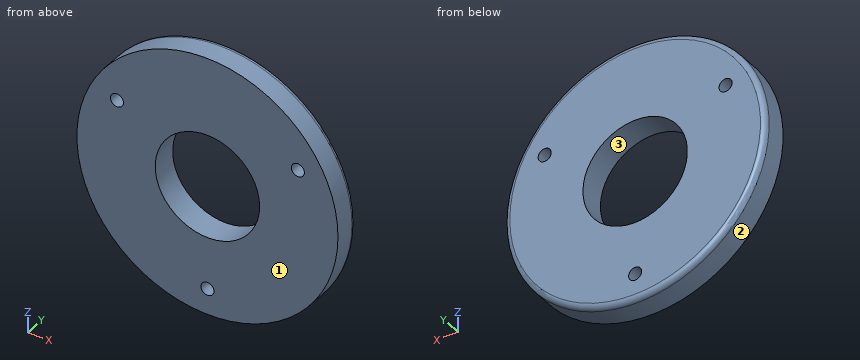
```python
from build123d import *

# Parameters (mm, degrees)
SKETCH1_R           = 63.5
BOSS_EXTRUDE1_DEPTH = 12.7
SKETCH2_R           = 25.4
CUT_EXTRUDE1_DEPTH  = 13.7
SKETCH3_R           = 3.175
CUT_EXTRUDE2_DEPTH  = 13.7
FILLET1_R           = 2.54


with BuildPart() as part:
    # Sketch1 → Boss-Extrude1 (new body)
    with BuildSketch(Plane(origin=(0, 0, 0), x_dir=(1, 0, 0), z_dir=(0, 1, 0))):
        Circle(SKETCH1_R)
    extrude(amount=BOSS_EXTRUDE1_DEPTH)

    # Sketch2 → Cut-Extrude1 (cut, through all)
    with BuildSketch(Plane(origin=(0, 12.7, 0), x_dir=(1, 0, 0), z_dir=(0, 1, 0))):
        Circle(SKETCH2_R)
    extrude(amount=-CUT_EXTRUDE1_DEPTH, mode=Mode.SUBTRACT)

    # Sketch3 → Cut-Extrude2 (cut, through all)
    with BuildSketch(Plane(origin=(0, 12.7, 0), x_dir=(1, 0, 0), z_dir=(0, 1, 0))):
        with Locations((0, 50.8)):
            Circle(SKETCH3_R)
        with Locations((43.994090512, -25.4)):
            Circle(SKETCH3_R)
        with Locations((-43.994090512, -25.4)):
            Circle(SKETCH3_R)
    extrude(amount=-CUT_EXTRUDE2_DEPTH, mode=Mode.SUBTRACT)

    # Fillet1
    fillet1_edges = [part.edges().sort_by_distance(p)[0] for p in [
        (-63.5, 12.7, 0),
    ]]
    fillet(fillet1_edges, radius=FILLET1_R)


solid = part.part
```
CAD build for the part. Positions are in the model's coordinates, mm. Face numbers are marked on the shaded views. Round coordinates to 2 decimals unless told otherwise and drop trailing zeros. Order: outer loops, then holes, each group sorted by start corner. A loop starts at its lowest first (then second) coordinate and runs counter-clockwise, first axis right, second up. Notation, with made-up numbers: (-4.75, 57.5) - (22.25, 57.5) arc R19 cw to (22.25, 91.5) - close; hole circle Ø11 at (-37, 10.5). An arc over 180 degrees is marked (long way). Answer in a Markdown table with one row per item. Add a question column.
(1) Probe L1, parallel to Z at x = 0, y = 9.25 (3 decimals); L2, parallel to Z at x = 1, y = 2; L3, parallel to X at y = 6.25, z = -14.5. List the from-to ranges inside material, lowest first. Write a range as [from, to].
(2) Drop flat-ended pins along their axis: pin 1 Ø5 at (x, y) = (5.5, 8.5) entering from +Z; pin 2 Ø5.5 at (x, z) = (0, -50.8) entering from -Y; pin 3 Ø3 at (x, y) = (41.5, 5.5) entering from -Z; pin 4 Ø1 at (x, y) = (-29, 4) entering from -Z. Give the stop position or say it passes through.
(3) Band-saw the part on A-A on x = 0. List the corners of the cut face in (y, z) (3 decimals).
(4) Band-saw the part on B-B on y = 2.75. List the corners of the cut face in (x, z) (3 decimals).
(5) Mould opens along Z. For the marked faces 1, 2 and 3 say: +Z half, -Z half, draft (parallel to the pull), parting line (faces both ways), or undercut.
Data:
| question | item | result |
|---|---|---|
| 1 | L1 | z = [-63.5, -53.975], [-47.625, -25.4], [25.4, 63.5] |
| 1 | L2 | z = [-63.49, -53.81], [-47.79, -25.38], [25.38, 63.49] |
| 1 | L3 | x = [-61.82, -20.85], [20.85, 61.82] |
| 2 | pin 1 | stops at z = 63.43 |
| 2 | pin 2 | passes through |
| 2 | pin 3 | stops at z = -49.32 |
| 2 | pin 4 | stops at z = -56.75 |
| 3 | outline | (0, -63.5) - (10.16, -63.5) arc R2.54 ccw to (12.7, -60.96) - (12.7, -53.975) - (0, -53.975) - close; (0, -47.625) - (12.7, -47.625) - (12.7, -25.4) - (0, -25.4) - close; (0, 25.4) - (12.7, 25.4) - (12.7, 60.96) arc R2.54 ccw to (10.16, 63.5) - (0, 63.5) - close |
| 4 | outline | circle Ø127 at (0, 0); hole circle Ø6.35 at (-43.994, 25.4); hole circle Ø50.8 at (0, 0); hole circle Ø6.35 at (0, -50.8); hole circle Ø6.35 at (43.994, 25.4) |
| 5 | face 1 | draft |
| 5 | face 2 | parting line |
| 5 | face 3 | undercut |
